```python
from build123d import *

# Parameters (mm, degrees)
EXTRUDE_1_DEPTH     = 1
SKETCH_2_R          = 0.75
CUT_EXTRUDE_1_DEPTH = 2
FILLET_1_R          = 1


with BuildPart() as part:
    # 草图1 → 凸台-拉伸1 (new body)
    with BuildSketch(Plane(origin=(0, 0, 0), x_dir=(1, 0, 0), z_dir=(0, 1, 0))):
        with BuildLine():
            Line((-4.5, -7.092954251), (-4.5, -10.092954251))
            Line((-4.5, -10.092954251), (-1.5, -10.734983296))
            Line((-1.5, -10.734983296), (-1.5, -6.734983296))
            ThreePointArc((-1.5, -6.734983296), (0, 6.9), (1.5, -6.734983296))
            Line((1.5, -6.734983296), (1.5, -10.734983296))
            Line((1.5, -10.734983296), (4.5, -10.092954251))
            Line((4.5, -10.092954251), (4.5, -7.092954251))
            ThreePointArc((4.5, -7.092954251), (0, 8.4), (-4.5, -7.092954251))
        make_face()
    extrude(amount=EXTRUDE_1_DEPTH)

    # 草图2 → 切除-拉伸1 (cut, through all)
    with BuildSketch(Plane(origin=(0, 1, 0), x_dir=(1, 0, 0), z_dir=(0, 1, 0))):
        with Locations((-3, -8.5)):
            Circle(SKETCH_2_R)
        with Locations((3, -8.5)):
            Circle(SKETCH_2_R)
    extrude(amount=-CUT_EXTRUDE_1_DEPTH, mode=Mode.SUBTRACT)

    # 圆角1
    fillet_1_edges = [part.edges().sort_by_distance(p)[0] for p in [
        (4.5, 0.5, 7.092954251),
        (4.5, 0.5, 10.092954251),
        (1.5, 0.5, 10.734983296),
        (-1.5, 0.5, 10.734983296),
        (-4.5, 0.5, 10.092954251),
        (-4.5, 0.5, 7.092954251),
    ]]
    fillet(fillet_1_edges, radius=FILLET_1_R)


solid = part.part
```
Design review of the part built by this model. Coordinates are the model's own, in mm. A direction names the side the tool comes from. Coordinates: 2 decimals unless noted, no trailing zeros. Loops run counter-clockwise (first coordinate to the right, second up) from the corner with the lowest first, then second, coordinate; pieces in that order, holes last.
Q1. Tool access review of faces 1 (the face through (1.5, 0.5, 8.1)), 2 (the face through (-4.5, 0.5, 8.4)), 3 (the face through (4.5, 0.5, 8.5)), 4 (the face through (2, 0, 7)): name each direction out of +Z, -Z, +X, -X, +Y, -Y from which nothing blocks a thin tool from reaching the whole face with its end or side.
Reported:
face 1: +Z, +Y, -Y
face 2: +Z, -X, +Y, -Y
face 3: +Z, +X, +Y, -Y
face 4: +Z, -Z, +X, -X, -Y
Q2. We need section A-A on y = 0.8. State the section outline as (x, z) points, and give its area (3 significant figures).
Reported:
outline: (-4.91, 6.81) arc R8.4 ccw (long way) to (4.91, 6.81) arc R1 cw to (4.5, 7.62) - (4.5, 9.28) arc R1 ccw to (3.71, 10.26) - (2.71, 10.48) arc R1 ccw to (1.5, 9.5) - (1.5, 6.73) arc R6.9 cw (long way) to (-1.5, 6.73) - (-1.5, 9.5) arc R1 ccw to (-2.71, 10.48) - (-3.71, 10.26) arc R1 ccw to (-4.5, 9.28) - (-4.5, 7.62) arc R1 cw to start; hole circle Ø1.5 at (-3, 8.5); hole circle Ø1.5 at (3, 8.5)
area: 78.9 mm2
Q3. We need section B-B on z = 0. State the section outline as (x, y) points, and give its area (3 significant figures).
Reported:
outline: (-8.4, 0) - (-6.9, 0) - (-6.9, 1) - (-8.4, 1) - close; (6.9, 0) - (8.4, 0) - (8.4, 1) - (6.9, 1) - close
area: 3.00 mm2
Q4. The part is to be moulded in two halves that separate along Z. For faces 5 (the face through (0.296, 0.493, -8.395)), 6 (the face through (2.45, 0.51, 7.99)), 7 (the face through (-1.5, 0.5, 8.1)), say which applies: +Z half, -Z half, draft (parallel to the pull), parting line (faces both ways), or undercut.
Reported:
face 5: parting line
face 6: undercut
face 7: draft
Q5. For pin 1 (0.5 mm diameter, centred on y = 0.5, z = 7.5, fed in from -X); pin 2 (0.5 mm diameter, centred on y = 0.5, z = 8.5, fed in from +X), all flat-tipped, find the tip position at first contact; note any pin that passes through.
Reported:
pin 1: stops at x = -4.57
pin 2: stops at x = 4.5
Q6. We need section C-C on x = -6. State the section outline as (y, z) points, and give its area (3 significant figures).
Reported:
outline: (0, -5.88) - (1, -5.88) - (1, -3.41) - (0, -3.41) - close; (0, 3.41) - (1, 3.41) - (1, 5.88) - (0, 5.88) - close
area: 4.94 mm2
Q7. We need section D-D on z = 8.5. State the section outline as (x, y) points.
Reported:
outline: (-4.5, 0) - (-3.75, 0) - (-3.75, 1) - (-4.5, 1) - close; (-2.25, 0) - (-1.5, 0) - (-1.5, 1) - (-2.25, 1) - close; (1.5, 0) - (2.25, 0) - (2.25, 1) - (1.5, 1) - close; (3.75, 0) - (4.5, 0) - (4.5, 1) - (3.75, 1) - close
Q8. To check wall thickness, follow line 1 (X direction, y = 0.75, z = 8.5); line 2 (Z direction, x = -3, y = 0.35); line 3 (X direction, y = 0.4, z = 0). State the ranges of each line that lie inside material, in increasing order.
Reported:
line 1: x = -4.5 to -3.75, -2.25 to -1.5, 1.5 to 2.25, 3.75 to 4.5
line 2: z = -7.85 to -6.21, 6.21 to 7.75, 9.25 to 10.41
line 3: x = -8.4 to -6.9, 6.9 to 8.4
